from build123d import *

# Parameters (mm, degrees)
F1_DEPTH = 260
F2_R     = 3.25
F3_DEPTH = 25
F4_SIZE  = 0.5


with BuildPart() as f1:
    # F0 (on Top) → F1 (new body, symmetric)
    with BuildSketch(Plane.XY):
        with BuildLine():
            Line((0, 12), (0, 1))
            ThreePointArc((0, 1), (-0.2928932188, 0.2928932188), (-1, 0))
            Line((-1, 0), (-100, 0))
            Line((-100, 0), (-100, -2))
            Line((-100, -2), (-1, -2))
            ThreePointArc((-1, -2), (1.1213203436, -1.1213203436), (2, 1))
            Line((2, 1), (2, 12))
            Line((2, 12), (0, 12))
        make_face()
    extrude(amount=F1_DEPTH, both=True)

    # F2 (on face) → F3 (cut)
    with BuildSketch(Plane.XZ.offset(2)):
        with Locations((-90, 252)):
            Circle(F2_R)
        with Locations((-90, -235)):
            Circle(F2_R)
        with Locations((-90, 92)):
            Circle(F2_R)
        with Locations((-90, -68)):
            Circle(F2_R)
    extrude(amount=-F3_DEPTH, mode=Mode.SUBTRACT)

    # F4
    f4_edges = [f1.edges().sort_by_distance(p)[0] for p in [
        (-93.25, -2, 252),
        (-86.75, -1, 252),
        (-93.25, 0, 252),
        (-93.25, -2, 92),
        (-86.75, -1, 92),
        (-93.25, 0, 92),
        (-93.25, -2, -68),
        (-86.75, -1, -68),
        (-93.25, 0, -68),
        (-93.25, -2, -235),
        (-86.75, -1, -235),
        (-93.25, 0, -235),
    ]]
    chamfer(f4_edges, length=F4_SIZE)


solid = f1.part
Verification items for the finished model (mm, model axes). A direction names the side the tool comes from. Coordinates: 2 decimals unless noted, no trailing zeros. Write each loop counter-clockwise with the first axis right and the second up, starting at its lowest first coordinate (ties: lowest second). Pieces come first, ordered by that corner, then holes. Notation, with made-up numbers: (26, -29) - (73, -29) arc R23 ccw to (73, 1) - close; hole circle Ø8 at (61.5, 12.5). An arc over 180 degrees is marked (long way). Answer as a JSON object with one key per item and string values.
(1) Gauge pin test, flat ends, axial feed: pin 1 Ø6 at (x, y) = (-37, 5.5) entering from +Z; pin 2 Ø8.5 at (x, z) = (-90, 252) entering from +Y. Record the tip position at first contact, or that the pin passes through.
Report:
{"pin 1": "through", "pin 2": "y = 0"}
(2) Cross-section at B-B on y = 5.5. Record the cut outline in (x, z), plus the area to 3 significant figures.
Report:
{"outline": "(0, -260) - (2, -260) - (2, 260) - (0, 260) - close", "area": "1,040 mm^2"}
(3) Tool access check on faces 1 (the flat face through (-51, -2, 4)), 2 (the flat face through (-50, 0, 4)). Record the directions out of +Z, -Z, +X, -X, +Y, -Y that give a thin tool (end or side, any length) a straight path to the whole face; none if there is none.
Report:
{"face 1": "+Z, -Z, +X, -X, -Y", "face 2": "+Z, -Z, -X, +Y"}
(4) Cross-section at A-A on z = 70. Record the cut outline in (x, y), plus the area to 3 significant figures.
Report:
{"outline": "(-100, -2) - (-1, -2) arc R3 ccw to (2, 1) - (2, 12) - (0, 12) - (0, 1) arc R1 cw to (-1, 0) - (-100, 0) - close", "area": "226 mm^2"}
(5) Cross-section at C-C on x = -79.5. Record the cut outline in (y, z), plus the area to 3 significant figures.
Report:
{"outline": "(-2, -260) - (0, -260) - (0, 260) - (-2, 260) - close", "area": "1,040 mm^2"}
(6) Thickness scan on line 1 along Z through (x, y) = (-90, -0.95); line 2 along Y through (x, z) = (-90, 119); line 3 along X through (y, z) = (1.25, 90). Record the ranges inside material, lowest first.
Report:
{"line 1": "-260 to -238.25, -231.75 to -71.25, -64.75 to 88.75, 95.25 to 248.75, 255.25 to 260", "line 2": "-2 to 0", "line 3": "0 to 2"}
